Geometry check sheet. Reference: the model listing, model coordinates, mm. A direction names the side the tool comes from. Round coordinates to 2 decimals unless told otherwise and drop trailing zeros. Write each loop counter-clockwise with the first axis right and the second up, starting at its lowest first coordinate (ties: lowest second). Pieces come first, ordered by that corner, then holes. Notation, with made-up numbers: (23.5, 79.25) - (63.5, 79.25) arc R26 cw to (63.5, 98.25) - close; hole circle Ø9 at (-2.5, 86). An arc over 180 degrees is marked (long way). Return JSON: item names as keys, results as strings.
```python
from build123d import *

# Parameters (mm, degrees)
SKETCH_1_R          = 3.75
SKETCH_1_R_2        = 2.25
EXTRUDE_1_DEPTH     = 2
SKETCH_2_R          = 3.75
SKETCH_2_R_2        = 2.5
EXTRUDE_2_DEPTH     = 1
EXTRUDE_START       = 2
SKETCH_3_R          = 3.75
SKETCH_3_R_2        = 2.5
EXTRUDE_3_DEPTH     = 2
SKETCH_4_R          = 1.5
SKETCH_4_R_2        = 1
CUT_EXTRUDE_1_DEPTH = 2
EXTRUDE_4_DEPTH     = 1
CUT_EXTRUDE_2_DEPTH = 1.1
CUT_EXTRUDE_4_DEPTH = 1.2


with BuildPart() as part:
    # 草图1 → 凸台-拉伸1 (new body)
    with BuildSketch(Plane(origin=(0, 0, 0), x_dir=(1, 0, 0), z_dir=(0, 1, 0))):
        Circle(SKETCH_1_R)
        with BuildLine():
            Line((16.2109375, 2.240090483), (0.3515625, 3.733484138))
            ThreePointArc((0.3515625, 3.733484138), (2.773162398, 2.524296003), (3.75, 0))
            ThreePointArc((3.75, 0), (2.773162398, -2.524296003), (0.3515625, -3.733484138))
            Line((0.3515625, -3.733484138), (16.2109375, -2.240090483))
            ThreePointArc((16.2109375, -2.240090483), (13.75, 0), (16.2109375, 2.240090483))
        make_face()
        with Locations((16, 0)):
            Circle(SKETCH_1_R_2)
    extrude(amount=EXTRUDE_1_DEPTH)

    # 草图2 → 凸台-拉伸2 (add)
    with BuildSketch(Plane(origin=(0, 2, 0), x_dir=(1, 0, 0), z_dir=(0, 1, 0))):
        with Locations(Location((0, 0, 0), (0, 0, 84.620621009))):
            Circle(SKETCH_2_R)
        with Locations(Location((0, 0, 0), (0, 0, 270))):
            Circle(SKETCH_2_R_2, mode=Mode.SUBTRACT)
    extrude(amount=EXTRUDE_2_DEPTH)

    # 草图3 → 凸台-拉伸3 (add)
    with BuildSketch(Plane.XZ.offset(EXTRUDE_START)):
        with Locations(Location((0, 0, 0), (0, 0, 270))):
            Circle(SKETCH_3_R)
        with Locations(Location((0, 0, 0), (0, 0, 90))):
            Circle(SKETCH_3_R_2, mode=Mode.SUBTRACT)
    extrude(amount=-EXTRUDE_3_DEPTH)

    # 草图4 → 切除-拉伸1 (cut)
    with BuildSketch(Plane(origin=(0, 2, 0), x_dir=(1, 0, 0), z_dir=(0, 1, 0))):
        with Locations(Location((0, 0, 0), (0, 0, 270))):
            Circle(SKETCH_4_R)
        with Locations(Location((4.92748738, 0, 0), (0, 0, 270))):
            Circle(SKETCH_4_R_2)
        with Locations(Location((7.92748738, 0, 0), (0, 0, 270))):
            Circle(SKETCH_4_R_2)
        with Locations(Location((10.92748738, 0, 0), (0, 0, 270))):
            Circle(SKETCH_4_R_2)
        with Locations(Location((13.92748738, 0, 0), (0, 0, 270))):
            Circle(SKETCH_4_R_2)
        with Locations(Location((16.92748738, 0, 0), (0, 0, 270))):
            Circle(SKETCH_4_R_2)
    extrude(amount=-CUT_EXTRUDE_1_DEPTH, mode=Mode.SUBTRACT)

    # 草图5 → 凸台-拉伸4 (add)
    with BuildSketch(Plane(origin=(0, 2, 0), x_dir=(1, 0, 0), z_dir=(0, 1, 0))):
        with BuildLine():
            Line((0.3515625, 3.733484138), (4.799205036, 3.31467311))
            Line((4.799205036, 3.31467311), (4.689652743, 2.151261914))
            Line((4.689652743, 2.151261914), (2.950077578, 2.315068527))
            ThreePointArc((2.950077578, 2.315068527), (1.796714366, 3.291552444), (0.3515625, 3.733484138))
        make_face()
        with BuildLine():
            Line((0.3515625, -3.733484138), (4.799205036, -3.31467311))
            Line((4.799205036, -3.31467311), (4.689652743, -2.258798299))
            Line((4.689652743, -2.258798299), (2.838244627, -2.450891151))
            ThreePointArc((2.838244627, -2.450891151), (1.71900511, -3.332794838), (0.3515625, -3.733484138))
        make_face()
    extrude(amount=EXTRUDE_4_DEPTH)

    # 草图6 → 切除-拉伸2 (cut)
    with BuildSketch(Plane(origin=(0.3515625, 0, 3.733484138), x_dir=(0.9955957701296245, 0, -0.09374999999999994), z_dir=(0.09374999999999994, 0, 0.9955957701296245))):
        Polygon((2.610250593, 3), (4.46731763, 2), (4.46731763, 3), align=None)
    extrude(amount=-CUT_EXTRUDE_2_DEPTH, mode=Mode.SUBTRACT)

    # 草图7 → 切除-拉伸4 (cut)
    with BuildSketch(Plane(origin=(0.3515625, 0, -3.733484138), x_dir=(-0.9955957701296245, 0, -0.09375), z_dir=(0.09375, 0, -0.9955957701296245))):
        Polygon((-2.586419937, 3), (-4.46731763, 2), (-4.46731763, 3), align=None)
    extrude(amount=-CUT_EXTRUDE_4_DEPTH, mode=Mode.SUBTRACT)


solid = part.part
```
(1) Section check D-D, the plane y = 0.6. Enter the section's corners in (x, z), plus the area to 3 significant figures.
Response values:
{"outline": "(0.35, -3.73) - (16.21, -2.24) arc R2.25 ccw to (16.21, 2.24) - (0.35, 3.73) arc R3.75 ccw (long way) to start; hole circle Ø3 at (0, 0); hole circle Ø2 at (4.93, 0); hole circle Ø2 at (7.93, 0); hole circle Ø2 at (10.93, 0); hole circle Ø2 at (13.93, 0); hole circle Ø2 at (16.93, 0)", "area": "104 mm^2"}
(2) Access from +Z, -Z, +X, -X, +Y, -Y to the whole of each face (thin tool, end or side, straight path). Record for faces 1 (the face through (0, 2, 2)), 2 (the face through (2.44, -1.01, -0.54)), 3 (the face through (3.79, 2.51, -2.82)).
Response values:
{"face 1": "+Y", "face 2": "-Y", "face 3": "+X, +Y"}
(3) Release check for a two-part mould opening along Z. For faces 4 (the face through (3, 3, 0)), 5 (the face through (12.95, 1.01, -0.22)), 6 (the face through (18.25, 0.99, 0.05)) record: pulls with the +Z half, pulls with the -Z half, needs draft (parallel to the pull), parting line crosses it, or undercut.
Response values:
{"face 4": "needs draft", "face 5": "undercut", "face 6": "parting line crosses it"}
(4) Material ranges on line 1 along X through (y, z) = (2.6, 0); line 2 along Z through (x, y) = (17, 0.75); line 3 along Y through (x, z) = (11, 2.5), recorded low to high. Write a range as [from, to].
Response values:
{"line 1": "x = [-3.75, -2.5], [2.5, 3.75]", "line 2": "z = [-2.02, -1], [1, 2.02]", "line 3": "y = [0, 2]"}
(5) Section check A-A, the plane x = 0. Enter the section's corners in (y, z).
Response values:
{"outline": "(-2, -3.75) - (3, -3.75) - (3, -2.5) - (2, -2.5) - (2, -1.5) - (0, -1.5) - (0, -2.5) - (-2, -2.5) - close; (-2, 2.5) - (0, 2.5) - (0, 1.5) - (2, 1.5) - (2, 2.5) - (3, 2.5) - (3, 3.75) - (-2, 3.75) - close"}
(6) Section check B-B, the plane y = -0.55. Enter the section's corners in (x, z).
Response values:
{"outline": "circle Ø7.5 at (0, 0); hole circle Ø5 at (0, 0)"}
(7) Gauge pin test, flat ends, axial feed: pin 1 (3 mm diameter, centred on x = 13.93, z = 0, fed in from -Y); pin 2 (3 mm diameter, centred on y = -0.5, z = -2, fed in from +X); pin 3 (4.5 mm diameter, centred on x = 0, z = 0, fed in from +Y). Record the tip position at first contact, or that the pin passes through.
Response values:
{"pin 1": "stops at y = 0", "pin 2": "stops at x = 18.17", "pin 3": "stops at y = 2"}
(8) Section check C-C, the plane z = 0. Give the number of separate pieces and of enclosed holes in the cut face, plus the area to 3 significant figures.
Response values:
{"separate pieces": "7", "enclosed holes": "0", "area": "25.5 mm^2"}
